from build123d import *

# Parameters (mm, degrees)
SKETCH1_R                = 0.75
BOSS_EXTRUDE1_DEPTH      = 10
BOSS_EXTRUDE2_DEPTH      = 1.5
BOSS_EXTRUDE2_DEPTH_BACK = 1.5


with BuildPart() as part:
    # Sketch1 → Boss-Extrude1 (new body)
    with BuildSketch(Plane(origin=(0, 0, 0), x_dir=(0, 0, -1), z_dir=(1, 0, 0))):
        Circle(SKETCH1_R)
    extrude(amount=BOSS_EXTRUDE1_DEPTH)

    # Sketch2 → Boss-Extrude2 (add, two sides: drawn at the far end of the back side and taken through both)
    with BuildSketch(Plane(origin=(0, 0, 0), x_dir=(1, 0, 0), z_dir=(0, 1, 0)).offset(-BOSS_EXTRUDE2_DEPTH_BACK)):
        Polygon((1, 1.75), (1, -1.75), (-4, -1.75), (-4, -0.75), (0, -0.75), (0, 0.75), (-4, 0.75), (-4, 1.75), align=None)
    extrude(amount=BOSS_EXTRUDE2_DEPTH + BOSS_EXTRUDE2_DEPTH_BACK)


solid = part.part
Check sheet for the modelled part. Datum: model origin and axes. Units: mm. A direction names the side the tool comes from. Give positions to 0.01 mm unless a question says otherwise; leave off trailing zeros. Loops run counter-clockwise (first coordinate to the right, second up) from the corner with the lowest first, then second, coordinate; pieces in that order, holes last. Notation, with made-up numbers: M 78.5,-19.5 L 122.5,-19.5 A22 cw 122.5,14.5 Z; hole C 61.5,38 d2. An arc over 180 degrees is marked long. Use a Markdown table: item, result. Add a question column.
Q1. Sectioned sample at B-B, the plane y = -0.9. Record the cut outline in (x, z), then the cut area to 3 significant figures.
Q2. Tool access check on faces 5 (the cylindrical face through (5.44, 0.03, 0.75)), 6 (the flat face through (-1, -1.5, -1)), 7 (the flat face through (0, 0, 0)). Record the directions out of +Z, -Z, +X, -X, +Y, -Y that give a thin tool (end or side, any length) a straight path to the whole face; none if there is none.
Q3. Sectioned sample at D-D, the plane y = 0. Record the cut outline in (x, z).
Q4. Mould release check, pull along Z, two halves, no side actions. Record for faces 1 (the flat face through (-2, 0, 0.75)), 2 (the flat face through (-4, 0, -1)), 3 (the flat face through (-1, 0, 1.75)), 4 (the flat face through (-2, 0, -1.75)): pulls with the +Z half, pulls with the -Z half, needs draft (parallel to the pull), parting line crosses it, or undercut.
Q5. Scan lines: line 1 along Z through (x, y) = (-3.25, -0.3); line 2 along X through (y, z) = (-0.1, -0.1); line 3 along X through (y, z) = (-0.1, 1). Record each from-to range of solid material in increasing order. Write a range as [from, to].
Q6. Sectioned sample at C-C, the plane z = 0.6. Record the cut outline in (x, y), then the cut area to 3 significant figures.
Q7. Sectioned sample at A-A, the plane x = -1.5. Record the cut outline in (y, z).
Verdict:
| question | item | result |
|---|---|---|
| 1 | outline | M -4,-1.75 L 1,-1.75 L 1,1.75 L -4,1.75 L -4,0.75 L 0,0.75 L 0,-0.75 L -4,-0.75 Z |
| 1 | area | 11.5 mm^2 |
| 2 | face 5 | +X |
| 2 | face 6 | +Z, -Z, +X, -X, -Y |
| 2 | face 7 | -X, +Y, -Y |
| 3 | outline | M -4,-1.75 L 1,-1.75 L 1,-0.75 L 10,-0.75 L 10,0.75 L 1,0.75 L 1,1.75 L -4,1.75 L -4,0.75 L 0,0.75 L 0,-0.75 L -4,-0.75 Z |
| 4 | face 1 | undercut |
| 4 | face 2 | needs draft |
| 4 | face 3 | pulls with the +Z half |
| 4 | face 4 | pulls with the -Z half |
| 5 | line 1 | [-1.75, -0.75], [0.75, 1.75] |
| 5 | line 2 | [0, 10] |
| 5 | line 3 | [-4, 1] |
| 6 | outline | M 0,-1.5 L 1,-1.5 L 1,-0.45 L 10,-0.45 L 10,0.45 L 1,0.45 L 1,1.5 L 0,1.5 Z |
| 6 | area | 11.1 mm^2 |
| 7 | outline | M -1.5,-1.75 L 1.5,-1.75 L 1.5,-0.75 L -1.5,-0.75 Z; M -1.5,0.75 L 1.5,0.75 L 1.5,1.75 L -1.5,1.75 Z |
